Source: CAD feature listing. Evaluate the final solid. Frame: model axes, mm. A direction names the side the tool comes from. Coordinates: 2 decimals unless noted, no trailing zeros. Write each loop counter-clockwise with the first axis right and the second up, starting at its lowest first coordinate (ties: lowest second). Pieces come first, ordered by that corner, then holes. Notation, with made-up numbers: M 10,25 L 69,25 A14 ccw 69,37 Z; hole C 15,1 d2. An arc over 180 degrees is marked long. One line per item, written item: value. Start each with the question number.
Item 1: Cut plane A-A, the plane x = -3. Output: boundary loops of the cut face in (y, z) (3 decimals), then the cut area to 3 significant figures.
Item 2: Pin query (flat end, axial travel): P1, Ø4, axis at x = -11.5, y = -35.5, coming from the +Z side; P2, Ø5, axis at x = -16.5, y = -13.5, coming from the +Z side; P3, Ø4, axis at x = -13, y = -9.5, coming from the -Z side. Return the tip coordinate at first contact, or that it passes through.
Item 3: Ray query, L1, parallel to Y at x = -1.5, z = 24.5; L2, parallel to Z at x = 7.5, y = -17.5; L3, parallel to Z at x = 17.5, y = -24. Return the intervals inside material, ascending. Write a range as from..to.
Item 4: Set-up query: faces 1 (the cylindrical face through (-20.87, -21.96, -65.08)), 2 (the flat face through (0, -29.984, 0)). Return all of +Z, -Z, +X, -X, +Y, -Y with unobstructed straight access to the full face (end or side cutting, diameter ignored); none if empty.
Item 5: Cut plane C-C, the plane y = -33. Output: boundary loops of the cut face in (x, z) (3 decimals).
Item 6: Cut plane B-B, the plane z = 27. Output: boundary loops of the cut face in (x, y) (3 decimals).
```python
from build123d import *

# Parameters (mm, degrees)
F1_DEPTH = 44.45
F2_R     = 3.175
F3_W     = 16.439201
F3_H     = 67.583382
F4_DEPTH = 50.801


with BuildPart() as f1:
    # F0 (on Front) → F1 (new body)
    with BuildSketch(Plane.XZ):
        with BuildLine():
            ThreePointArc((25.4, 53.975), (20.75032, 65.20032), (9.525, 69.85))
            Line((9.525, 69.85), (-9.525, 69.85))
            ThreePointArc((-9.525, 69.85), (-20.75032, 65.20032), (-25.4, 53.975))
            Line((-25.4, 53.975), (-25.4, -53.975))
            ThreePointArc((-25.4, -53.975), (-20.75032, -65.20032), (-9.525, -69.85))
            Line((-9.525, -69.85), (9.525, -69.85))
            ThreePointArc((9.525, -69.85), (20.75032, -65.20032), (25.4, -53.975))
            Line((25.4, -53.975), (25.4, 53.975))
        make_face()
    extrude(amount=F1_DEPTH)

    # F2
    f2_edges = [f1.edges().sort_by_distance(p)[0] for p in [
        (20.75032, -44.45, 65.20032),
        (20.75032, 0, 65.20032),
    ]]
    fillet(f2_edges, radius=F2_R)

    # F3 (on face) → F4 (cut, through all)
    with BuildSketch(Plane.YZ.offset(25.4)):
        with Locations((-21.764164, 0)):
            Rectangle(F3_W, F3_H)
    extrude(amount=-F4_DEPTH, mode=Mode.SUBTRACT)


solid = f1.part
```
From the geometry:
1. outline: M -44.45,-66.675 A3.175 ccw -41.275,-69.85 L -3.175,-69.85 A3.175 ccw 0,-66.675 L 0,66.675 A3.175 ccw -3.175,69.85 L -41.275,69.85 A3.175 ccw -44.45,66.675 Z; hole M -29.984,-33.792 L -13.545,-33.792 L -13.545,33.792 L -29.984,33.792 Z
1. area: 5,090 mm²
2. P1: stops at z = 69.85
2. P2: stops at z = 69.21
2. P3: stops at z = -69.78
3. L1: y = -44.45..-29.98, -13.54..0
3. L2: z = -69.85..-33.79, 33.79..69.85
3. L3: z = -67.7..-33.79, 33.79..67.7
4. face 1: -Z, -X, +Y, -Y
4. face 2: +X, -X
5. outline: M -25.4,-53.975 A15.875 ccw -9.525,-69.85 L 9.525,-69.85 A15.875 ccw 25.4,-53.975 L 25.4,53.975 A15.875 ccw 9.525,69.85 L -9.525,69.85 A15.875 ccw -25.4,53.975 Z
6. outline: M -25.4,-41.275 A3.175 ccw -22.225,-44.45 L 22.225,-44.45 A3.175 ccw 25.4,-41.275 L 25.4,-29.984 L -25.4,-29.984 Z; M -25.4,-13.545 L 25.4,-13.545 L 25.4,-3.175 A3.175 ccw 22.225,0 L -22.225,0 A3.175 ccw -25.4,-3.175 Z
